```python
from build123d import *

# Parameters (mm, degrees)
DODANIE_WYCI_GNI_CIE1_DEPTH = 5.2
SZKIC3_W                    = 60
SZKIC3_H                    = 159.9
SZKIC5_W                    = 99.9
SZKIC5_H                    = 199.8
SZKIC6_W                    = 49.271239353
SZKIC6_H                    = 120
WYTNIJ_WYCI_GNI_CIE1_DEPTH  = 78
WYTNIJ_WYCI_GNI_CIE2_DEPTH  = 5.6
SZKIC9_R                    = 2.424871131
SZKIC9_R_2                  = 1.2
DODANIE_WYCI_GNI_CIE3_DEPTH = 3.8
SZKIC10_W                   = 50
SZKIC10_H                   = 39.9
WYTNIJ_WYCI_GNI_CIE4_DEPTH  = 24
DODANIE_WYCI_GNI_CIE4_DEPTH = 50


with BuildPart() as part:
    # Szkic2 → Dodanie-wyciągnięcie1 (new body)
    with BuildSketch(Plane.XY):
        Polygon((18.542832418, 83.245366469), (18.542832418, 43.345366469), (-51.457167582, 43.345366469), (-51.457167582, -76.654633531), (18.542832418, -76.654633531), (18.542832418, -116.554633531), (-81.357167582, -116.554633531), (-81.357167582, 83.245366469), align=None)
    extrude(amount=DODANIE_WYCI_GNI_CIE1_DEPTH)

    # Szkic3 → Wyciągnięcie po profilach3 section 0
    with BuildSketch(Plane.XY.offset(11.5)):
        with Locations((-11.457167582, 3.295366469)):
            Rectangle(SZKIC3_W, SZKIC3_H)
    # Szkic5 → Wyciągnięcie po profilach3 section 1
    with BuildSketch(Plane.XY.offset(5.2)):
        with Locations((-31.407167582, -16.654633531)):
            Rectangle(SZKIC5_W, SZKIC5_H)
    loft()

    # Szkic6 → Wytnij-wyciągnięcie1 (cut)
    with BuildSketch(Plane(origin=(-51.457167582, 0, 0), x_dir=(0, 0, -1), z_dir=(1, 0, 0))):
        with Locations((-24.635619677, -16.654633531)):
            Rectangle(SZKIC6_W, SZKIC6_H)
    extrude(amount=WYTNIJ_WYCI_GNI_CIE1_DEPTH, mode=Mode.SUBTRACT)

    # Szkic7 → Wytnij-wyciągnięcie2 (cut)
    with BuildSketch(Plane(origin=(-51.457167582, 0, 0), x_dir=(0, 0, -1), z_dir=(1, 0, 0))):
        Polygon((-5.12, -34.1297624), (-7.22, -35.342197966), (-7.22, -37.767069096), (-5.12, -38.979504662), (-3.02, -37.767069096), (-3.02, -35.342197966), align=None)
        Polygon((-5.12, 5.6702376), (-7.22, 4.457802034), (-7.22, 2.032930904), (-5.12, 0.820495338), (-3.02, 2.032930904), (-3.02, 4.457802034), align=None)
    extrude(amount=-WYTNIJ_WYCI_GNI_CIE2_DEPTH, mode=Mode.SUBTRACT)

    # Szkic9 → Dodanie-wyciągnięcie3 (add)
    with BuildSketch(Plane(origin=(-51.457167582, 0, 0), x_dir=(0, 0, -1), z_dir=(1, 0, 0))):
        with Locations((-5.12, 3.245366469)):
            Circle(SZKIC9_R)
        with Locations((-5.12, 3.245366469)):
            Circle(SZKIC9_R_2, mode=Mode.SUBTRACT)
        with Locations((-5.12, -36.554633531)):
            Circle(SZKIC9_R)
        with Locations((-5.12, -36.554633531)):
            Circle(SZKIC9_R_2, mode=Mode.SUBTRACT)
    extrude(amount=-DODANIE_WYCI_GNI_CIE3_DEPTH)

    # Szkic10 → Wytnij-wyciągnięcie4 (cut)
    with BuildSketch(Plane.XY.offset(11.5)):
        with Locations((-6.457167582, 63.295366469)):
            Rectangle(SZKIC10_W, SZKIC10_H)
    extrude(amount=-WYTNIJ_WYCI_GNI_CIE4_DEPTH, mode=Mode.SUBTRACT)


with BuildPart() as body_2:
    # Lustro1: mirrored copy
    add(part.part.mirror(Plane(origin=(18.542832418, 83.245366469, 5.2), x_dir=(0, 0, 1), z_dir=(-1, 0, 0))))


with BuildPart() as body_2_1:
    # Obiekt-Przenieś/Kopiuj1: moved
    add(body_2.part.moved(Location((34.890139481, 0, 0))))

    # Szkic11 → Dodanie-wyciągnięcie4 (add)
    with BuildSketch(Plane.ZY.offset(-53.432971899)):
        Polygon((11.5, -76.654633531), (1.5, -76.654633531), (10.5, -66.654633531), (11.5, -66.654633531), align=None)
    extrude(amount=-DODANIE_WYCI_GNI_CIE4_DEPTH)


solid = body_2_1.part
```
Verification items for the finished model (mm, model axes). A direction names the side the tool comes from. Coordinates: 2 decimals unless noted, no trailing zeros. Put each result on its own line as item: value. Start each with the question number.
1) Tool access check on faces 1 (the flat face through (114, 43.345, 6)), 2 (the flat face through (103.433, 63, 6)), 3 (the flat face through (104, -76.655, 5)), 4 (the flat face through (127.233, -38, 6)), 5 (the flat face through (103.433, -73, 8)). Record the directions out of +Z, -Z, +X, -X, +Y, -Y that give a thin tool (end or side, any length) a straight path to the whole face; none if there is none.
2) Go/stop test with flat-tipped pins: pin 1 (2 mm diameter, centred on x = 127.5, y = -36.5, fed in from +Z); pin 2 (3 mm diameter, centred on y = -20.5, z = 5, fed in from -X); pin 3 (0.5 mm diameter, centred on x = 128, y = 3, fed in from +Z). Record where each tip stops, or that it passes through.
3) Material ranges on L1, parallel to Y at x = 126.1, z = 5.12; L2, parallel to X at y = 26.5, z = 1; L3, parallel to Z at x = 140, y = 16.5, recorded low to high.
4) Release check for a two-part mould opening along Y. For faces 6 (the flat face through (78.08, -71.72, 5.94)), 7 (the flat face through (129.033, -37, 5)), 8 (the flat face through (53.433, -91, 5)) record: pulls with the +Y half, pulls with the -Y half, needs draft (parallel to the pull), parting line crosses it, or undercut.
Geometry check:
1. face 1: +Z, -Z, -X
1. face 2: +Z, -Z, -X, +Y
1. face 3: -Z
1. face 4: none
1. face 5: +Z, -Z
2. pin 1: stops at z = 9.44
2. pin 2: stops at x = 123.43
2. pin 3: stops at z = 9.24
3. L1: y = -116.55 to -37.75, -35.35 to 2.05, 4.45 to 83.25
3. L2: x = 123.43 to 153.33
3. L3: z = 0 to 7.31
4. face 6: pulls with the +Y half
4. face 7: undercut
4. face 8: needs draft
